Read the model definition and answer for the solid it produces. Units are mm, in the model's axes. A direction names the side the tool comes from. Coordinates: 2 decimals unless noted, no trailing zeros. Order: outer loops, then holes, each group sorted by start corner. A loop starts at its lowest first (then second) coordinate and runs counter-clockwise, first axis right, second up. Notation, with made-up numbers: (29.5, 85) -> (66.5, 85) arc R28 ccw to (66.5, 116) -> close; hole circle Ø11 at (15, 44). An arc over 180 degrees is marked (long way). Answer in a Markdown table with one row per item.
from build123d import *


with BuildPart() as part:
    # Sketch1 → Revolve4 (revolve)
    with BuildSketch(Plane(origin=(0, 0, 0), x_dir=(0, 0, -1), z_dir=(1, 0, 0))):
        with BuildLine():
            Line((50, 13), (50, 11))
            ThreePointArc((50, 11), (49.853553391, 10.646446609), (49.5, 10.5))
            Line((49.5, 10.5), (0, 10.5))
            Line((0, 10.5), (0, 9.5))
            Line((0, 9.5), (50.5, 9.5))
            ThreePointArc((50.5, 9.5), (50.853553391, 9.646446609), (51, 10))
            Line((51, 10), (51, 12))
            ThreePointArc((51, 12), (51.146446609, 12.353553391), (51.5, 12.5))
            Line((51.5, 12.5), (80, 12.5))
            Line((80, 12.5), (80, 13.5))
            Line((80, 13.5), (50.5, 13.5))
            ThreePointArc((50.5, 13.5), (50.146446609, 13.353553391), (50, 13))
        make_face()
    revolve(axis=Axis((0, 0, 0), (0, 0, -1)))


solid = part.part
Q1. For a pull along Y with two mould halves and no side action, classify faces 1 (the face through (-13.18, -2.93, -65.04)), 2 (the face through (3.755, 11.923, -65.95)), 3 (the face through (-9, -9, -80)) as pulls with the +Y half, pulls with the -Y half, needs draft (parallel to the pull), parting line crosses it, or undercut.
Outcome:
| item | result |
|---|---|
| face 1 | parting line crosses it |
| face 2 | undercut |
| face 3 | needs draft |
Q2. The part is cut by section A-A (y = 0). Write down the section's boundary in (x, z), then the cut area to 3 significant figures.
Outcome:
| item | result |
|---|---|
| outline | (-13.5, -80) -> (-12.5, -80) -> (-12.5, -51.5) arc R0.5 cw to (-12, -51) -> (-10, -51) arc R0.5 ccw to (-9.5, -50.5) -> (-9.5, 0) -> (-10.5, 0) -> (-10.5, -49.5) arc R0.5 cw to (-11, -50) -> (-13, -50) arc R0.5 ccw to (-13.5, -50.5) -> close; (9.5, -50.5) arc R0.5 ccw to (10, -51) -> (12, -51) arc R0.5 cw to (12.5, -51.5) -> (12.5, -80) -> (13.5, -80) -> (13.5, -50.5) arc R0.5 ccw to (13, -50) -> (11, -50) arc R0.5 cw to (10.5, -49.5) -> (10.5, 0) -> (9.5, 0) -> close |
| area | 166 mm² |
Q3. Given pin 1 (3 mm diameter, centred on x = 5, y = -7.5, fed in from -Z); pin 2 (10 mm diameter, centred on y = 6.5, z = -26.5, fed in from -X); pin 3 (12 mm diameter, centred on x = -3, y = -1.5, fed in from -Z); pin 4 (10 mm diameter, centred on y = 5, z = -24, fed in from +X), each flat-ended and moving along its own axis, determine where each tip first touches the part or whether it passes through.
Outcome:
| item | result |
|---|---|
| pin 1 | z = -51 |
| pin 2 | x = -10.39 |
| pin 3 | through |
| pin 4 | x = 10.5 |
Q4. The part is cut by section C-C (z = -65). Write down the section's boundary in (x, y), then the cut area to 3 significant figures.
Outcome:
| item | result |
|---|---|
| outline | circle Ø27 at (0, 0); hole circle Ø25 at (0, 0) |
| area | 81.7 mm² |
Q5. For faces 4 (the face through (-9, -5, 0)), 5 (the face through (9, 5, -51)), 6 (the face through (3.2, 10, -24.4)), determine the directions among +Z, -Z, +X, -X, +Y, -Y from which every point of the face is accessible in a straight line to the end or side of a thin tool.
Outcome:
| item | result |
|---|---|
| face 4 | +Z, +X, -X, +Y, -Y |
| face 5 | -Z |
| face 6 | +Z |
Q6. Consider line 1 (X direction, y = 0, z = -74); line 2 (X direction, y = 0, z = -21); line 3 (Y direction, x = 0.5, z = -7). Determine where each line is inside the solid, lowest interval first.
Outcome:
| item | result |
|---|---|
| line 1 | -13.5 to -12.5, 12.5 to 13.5 |
| line 2 | -10.5 to -9.5, 9.5 to 10.5 |
| line 3 | -10.49 to -9.49, 9.49 to 10.49 |
